```python
from build123d import *

# Parameters (mm, degrees)
SKETCH_3_W               = 80
SKETCH_3_H               = 110
EXTRUDE_2_DEPTH          = 20
SKETCH_4_W               = 60
SKETCH_4_H               = 70
EXTRUDE_3_DEPTH          = 70
SKETCH_5_W               = 10
SKETCH_5_H               = 110
EXTRUDE_4_DEPTH          = 50
SKETCH_6_W               = 20
SKETCH_6_H               = 40
CUT_EXTRUDE_1_DEPTH      = 98.59610648
CUT_EXTRUDE_2_DEPTH      = 98.59610648
CUT_EXTRUDE_3_DEPTH      = 98.59610648
CUT_EXTRUDE_3_DEPTH_BACK = 98.59610648
SKETCH_8_R               = 25


with BuildPart() as part:
    # Эскиз3 → Бобышка-Вытянуть2 (new body)
    with BuildSketch(Plane(origin=(0, 0, 0), x_dir=(1, 0, 0), z_dir=(0, 1, 0))):
        Rectangle(SKETCH_3_W, SKETCH_3_H)
    extrude(amount=EXTRUDE_2_DEPTH)

    # Эскиз4 → Бобышка-Вытянуть3 (add)
    with BuildSketch(Plane(origin=(0, 0, 0), x_dir=(1, 0, 0), z_dir=(0, 1, 0))):
        with Locations((-10, 0)):
            Rectangle(SKETCH_4_W, SKETCH_4_H)
    extrude(amount=EXTRUDE_3_DEPTH)

    # Эскиз5 → Бобышка-Вытянуть4 (add)
    with BuildSketch(Plane(origin=(0, 0, 0), x_dir=(1, 0, 0), z_dir=(0, 1, 0))):
        with Locations((-35, 0)):
            Rectangle(SKETCH_5_W, SKETCH_5_H)
    extrude(amount=EXTRUDE_4_DEPTH)

    # Эскиз6 → Вырез-Вытянуть1 (cut, through all)
    with BuildSketch(Plane(origin=(0, 0, 0), x_dir=(1, 0, 0), z_dir=(0, 1, 0))):
        with Locations((30, 0)):
            Rectangle(SKETCH_6_W, SKETCH_6_H)
    extrude(amount=CUT_EXTRUDE_1_DEPTH, mode=Mode.SUBTRACT)

    # Эскиз7 → Вырез-Вытянуть2 (cut, through all)
    with BuildSketch(Plane(origin=(0, 0, 0), x_dir=(0, 0, -1), z_dir=(1, 0, 0))):
        Polygon((-55, 20), (-35, 50), (-55, 50), align=None)
        Polygon((55, 20), (35, 50), (55, 50), align=None)
    extrude(amount=-CUT_EXTRUDE_2_DEPTH, mode=Mode.SUBTRACT)

    # Эскиз8 → Вырез-Вытянуть3 (cut, two sides: drawn at the far end of the back side and taken through both)
    with BuildSketch(Plane(origin=(0, 0, 0), x_dir=(0, 0, -1), z_dir=(1, 0, 0)).offset(-CUT_EXTRUDE_3_DEPTH_BACK)):
        with Locations((0, 70)):
            Circle(SKETCH_8_R)
    extrude(amount=CUT_EXTRUDE_3_DEPTH + CUT_EXTRUDE_3_DEPTH_BACK, mode=Mode.SUBTRACT)


solid = part.part
```
Build history of the part. All positions in model axes, mm. A direction names the side the tool comes from. Round coordinates to 2 decimals unless told otherwise and drop trailing zeros. Loops run counter-clockwise (first coordinate to the right, second up) from the corner with the lowest first, then second, coordinate; pieces in that order, holes last. Notation, with made-up numbers: M 15,78 L 32,78 A17 cw 32,104 Z; hole C 51.5,20.25 d5. An arc over 180 degrees is marked long. Answer as CSV lines item,"result".
1. Cut at B-B on z = -43.5. Write the cut outline in (x, y), then the cut area to 3 significant figures.
Resolved:
outline,"M -40,0 L 40,0 L 40,20 L -30,20 L -30,37.25 L -40,37.25 Z"
area,"1,770 mm²"
2. Cut at C-C on y = 17. Write the cut outline in (x, z), then the cut area to 3 significant figures.
Resolved:
outline,"M -40,-55 L 40,-55 L 40,-20 L 20,-20 L 20,20 L 40,20 L 40,55 L -40,55 Z"
area,"8,000 mm²"
3. Flat gauge pins, fed straight in: P1, Ø21, axis at y = 25, z = -3.5, coming from the +X side; P2, Ø1, axis at x = 12, z = 0, coming from the +Y side (3 decimals); P3, Ø10, axis at x = 19, z = 3, coming from the +Y side; P4, Ø3, axis at y = 51, z = -36, coming from the -X side. Where does each tip first touch, or does it go through?
Resolved:
P1,"stops at x = 20"
P2,"stops at y = 45.005"
P3,"stops at y = 46.31"
P4,"stops at x = -40"
4. Cut at D-D on x = -5.5. Write the cut outline in (y, z).
Resolved:
outline,"M 0,-55 L 20,-55 L 20,-35 L 70,-35 L 70,-25 A25 cw 70,25 L 70,35 L 20,35 L 20,55 L 0,55 Z"
5. Two-plate mould, pull along Z, no slides. Class faces 6 (the cylindrical face through (-10.42, 45.006, 0.55)), 7 (the flat face through (-40, 27, 1)), 8 (the flat face through (-1, 10, -55)), 9 (the flat face through (20, 35, 0)): released by +Z, released by -Z, zero draft, split by the parting line, or undercut.
Resolved:
face 6,"undercut"
face 7,"zero draft"
face 8,"released by -Z"
face 9,"undercut"
6. 3-axis set-ups, long thin cutter, end or side, ignore diameter. For faces 1 (the flat face through (-35, 35, 45)), 2 (the flat face through (-30, 28, 41)), 3 (the flat face through (40, 10, -37)), 4 (the flat face through (30, 10, -20)), 5 (the flat face through (-10, 45, -35)): which of +Z, -Z, +X, -X, +Y, -Y reach the whole face in a straight line?
Resolved:
face 1,"+Z, +X, -X, +Y"
face 2,"+Z, +X, +Y"
face 3,"+Z, -Z, +X, +Y, -Y"
face 4,"+X, +Y, -Y"
face 5,"-Z, +X, +Y"
7. Cut at A-A on x = 30.5. Write the cut outline in (y, z), then the cut area to 3 significant figures.
Resolved:
outline,"M 0,-55 L 20,-55 L 20,-20 L 0,-20 Z; M 0,20 L 20,20 L 20,55 L 0,55 Z"
area,"1,400 mm²"
8. Wall check: probe 1 along Z at (x, y) = (27, 9); probe 2 along Z at (x, y) = (0, 26.5); probe 3 along Z at (x, y) = (4, 57.5). Give the ranges that are in metal, low to high. Write a range as [from, to].
Resolved:
probe 1,"z = [-55, -20], [20, 55]"
probe 2,"z = [-35, 35]"
probe 3,"z = [-35, -21.65], [21.65, 35]"
